For this review, use the dimensioned drawing (mm, ordinates from the lowest corner) and the shaded views. Coordinates: 2 decimals unless noted, no trailing zeros. Order: outer loops, then holes, each group sorted by start corner. A loop starts at its lowest first (then second) coordinate and runs counter-clockwise, first axis right, second up. Notation, with made-up numbers: M 30,-30.75 L 78,-30.75 A36 cw 78,4.25 Z; hole C 88,-16.5 d9. An arc over 180 degrees is marked long. Use CSV: the item, a comma, the result in double quotes.
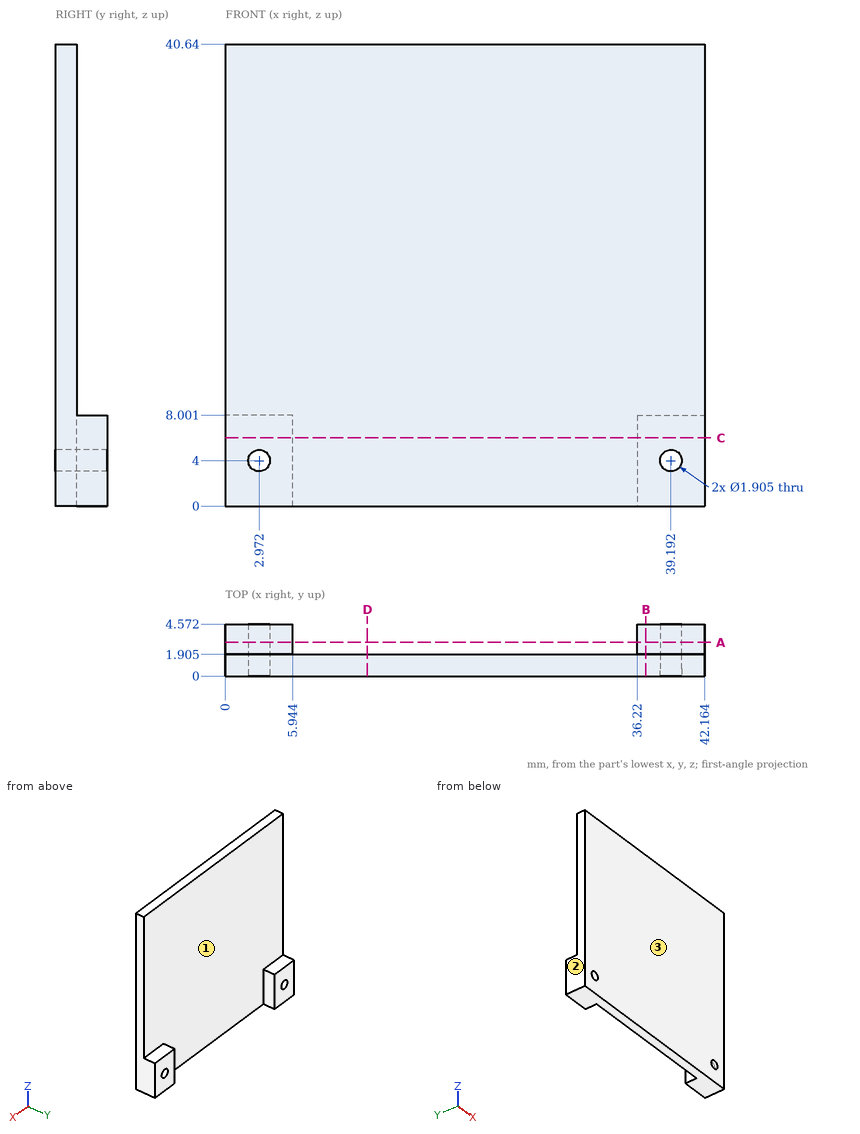
Item 1: Clearance check with flat-ended pins moving along their axes: pin 1 Ø2 at (x, y) = (39, 3) entering from +Z; pin 2 Ø2 at (y, z) = (4, 20) entering from +X; pin 3 Ø2 at (x, z) = (13, 13.5) entering from +Y (1 decimal). State where each tip first meets the part, or that it passes through.
Solutions:
pin 1,"z = 8"
pin 2,"through"
pin 3,"y = 1.9"
Item 2: Add section A-A on y = 2.95. State the section outline as (x, z) points (1 decimal).
Solutions:
outline,"M 0,0 L 5.9,0 L 5.9,8 L 0,8 Z; M 36.2,0 L 42.2,0 L 42.2,8 L 36.2,8 Z; hole C 3,4 d1.9; hole C 39.2,4 d1.9"
Item 3: Add section B-B on x = 37. State the section outline as (y, z) points (1 decimal).
Solutions:
outline,"M 0,0 L 4.6,0 L 4.6,8 L 1.9,8 L 1.9,40.6 L 0,40.6 Z"
Item 4: Add section D-D on x = 12.5. State the section outline as (y, z) points (1 decimal).
Solutions:
outline,"M 0,0 L 1.9,0 L 1.9,40.6 L 0,40.6 Z"
Item 5: To check wall thickness, follow line 1 along Y through (x, z) = (33.5, 21) (1 decimal); line 2 along X through (y, z) = (2.4, 6) (1 decimal); line 3 along Z through (x, y) = (38.5, 2.1) (1 decimal). State the ranges of each line that lie inside material, in increasing order. Write a range as [from, to].
Solutions:
line 1,"[0, 1.9]"
line 2,"[0, 5.9], [36.2, 42.2]"
line 3,"[0, 3.3], [4.7, 8]"
Item 6: Draft analysis for pull direction X (two halves, no side actions). For the marked faces 1, 2 and 3, state which applies: released by +X, released by -X, zero draft, split by the parting line, or undercut.
Solutions:
face 1,"undercut"
face 2,"released by -X"
face 3,"zero draft"
Item 7: Add section C-C on z = 6. State the section outline as (x, y) points (1 decimal).
Solutions:
outline,"M 0,0 L 42.2,0 L 42.2,4.6 L 36.2,4.6 L 36.2,1.9 L 5.9,1.9 L 5.9,4.6 L 0,4.6 Z"
